from build123d import *

# Parameters (mm, degrees)
BOSS_EXTRUDE1_DEPTH = 10
SKETCH2_R           = 2.7
CUT_EXTRUDE1_DEPTH  = 53.440442409
SKETCH3_R           = 2.7
CUT_EXTRUDE2_DEPTH  = 34.541019662
FILLET1_R           = 2


with BuildPart() as part:
    # Sketch1 → Boss-Extrude1 (new body)
    with BuildSketch(Plane(origin=(0, 0, 0), x_dir=(1, 0, 0), z_dir=(0, 1, 0))):
        Polygon((-25, 0), (25, 0), (25, -5), (-20, -5), (-20, -25), (-25, -25), align=None)
    extrude(amount=BOSS_EXTRUDE1_DEPTH)

    # Sketch2 → Cut-Extrude1 (cut, through all)
    with BuildSketch(Plane(origin=(-20, 0, 0), x_dir=(0, 0, -1), z_dir=(1, 0, 0))):
        with Locations((-19.4, 4.4)):
            Circle(SKETCH2_R)
    extrude(amount=-CUT_EXTRUDE1_DEPTH, mode=Mode.SUBTRACT)

    # Sketch3 → Cut-Extrude2 (cut, through all)
    with BuildSketch(Plane.XY.offset(5)):
        with Locations((19.4, 4.4)):
            Circle(SKETCH3_R)
    extrude(amount=-CUT_EXTRUDE2_DEPTH, mode=Mode.SUBTRACT)

    # Fillet1
    fillet1_edges = [part.edges().sort_by_distance(p)[0] for p in [
        (-20, 5, 5),
    ]]
    fillet(fillet1_edges, radius=FILLET1_R)


solid = part.part
Input: part model. Units: mm. Frame: model coordinates. A direction names the side the tool comes from. Give positions to 0.01 mm unless a question says otherwise; leave off trailing zeros. Order: outer loops, then holes, each group sorted by start corner. A loop starts at its lowest first (then second) coordinate and runs counter-clockwise, first axis right, second up. Notation, with made-up numbers: M 26.5,29.25 L 78.5,29.25 A7 cw 78.5,33.25 Z; hole C 81,-9 d8. An arc over 180 degrees is marked long. Answer as a JSON object with one key per item and string values.
1. Reachability of faces 4 (the flat face through (-25, 5, 13)), 5 (the flat face through (4, 5, 5)) from +Z, -Z, +X, -X, +Y, -Y: full face, straight path, thin tool, end or side. Return the list, or none.
Result sheet:
{"face 4": "+Z, -Z, -X, +Y, -Y", "face 5": "+Z, +X, +Y, -Y"}
2. Pull-direction query (Y, two-part tool) for faces 1 (the flat face through (-7, 10, 4)), 2 (the flat face through (-20, 5, 16)), 3 (the cylindrical face through (20.852, 6.677, 2.535)); classes: +Y half, -Y half, draft (parallel to the pull), parting line (faces both ways), or undercut.
Result sheet:
{"face 1": "+Y half", "face 2": "draft", "face 3": "undercut"}
3. Cut plane D-D, the plane y = 8.5. Output: boundary loops of the cut face in (x, z).
Result sheet:
{"outline": "M -25,0 L 25,0 L 25,5 L -18,5 A2 cw -20,7 L -20,25 L -25,25 Z"}
4. Cut plane C-C, the plane z = 19.4. Output: boundary loops of the cut face in (x, y), and give its area (3 significant figures).
Result sheet:
{"outline": "M -25,0 L -20,0 L -20,1.7 L -25,1.7 Z; M -25,7.1 L -20,7.1 L -20,10 L -25,10 Z", "area": "23.0 mm²"}
5. First-contact query: P1, Ø1.5, axis at x = -11.5, y = 5, coming from the +Z side; P2, Ø5, axis at y = 4.4, z = 19.4, coming from the -X side; P3, Ø3, axis at y = 6.5, z = 18.5, coming from the +X side. Flat tips, straight axial feed; report the tip coordinate or a pass-through.
Result sheet:
{"P1": "z = 5", "P2": "through", "P3": "x = -20"}
6. Ray query, line 1 (Y direction, x = 19.4, z = 3.8); line 2 (X direction, y = 7.5, z = 13); line 3 (Z direction, x = 1.5, y = 6). Return the intervals inside material, ascending. Write a range as [from, to].
Result sheet:
{"line 1": "[0, 1.7], [7.1, 10]", "line 2": "[-25, -20]", "line 3": "[0, 5]"}
7. Cut plane A-A, the plane x = 19.4. Output: boundary loops of the cut face in (y, z), and give its area (3 significant figures).
Result sheet:
{"outline": "M 0,0 L 1.7,0 L 1.7,5 L 0,5 Z; M 7.1,0 L 10,0 L 10,5 L 7.1,5 Z", "area": "23.0 mm²"}
8. Cut plane B-B, the plane y = 4.4. Output: boundary loops of the cut face in (x, z).
Result sheet:
{"outline": "M -25,0 L 16.7,0 L 16.7,5 L -18,5 A2 cw -20,7 L -20,16.7 L -25,16.7 Z; M -25,22.1 L -20,22.1 L -20,25 L -25,25 Z; M 22.1,0 L 25,0 L 25,5 L 22.1,5 Z"}
